Input: part model. Units: mm. Frame: model coordinates. Face numbers are marked on the shaded views. Give positions to 0.01 mm unless a question says otherwise; leave off trailing zeros. Loops run counter-clockwise (first coordinate to the right, second up) from the corner with the lowest first, then second, coordinate; pieces in that order, holes last. Notation, with made-up numbers: (47, 78) - (97, 78) arc R10 ccw to (97, 96) - close; hole circle Ø2 at (-15.75, 59.25). An arc over 180 degrees is marked (long way). Answer as a JSON object with one key per item and string values. Group by question number.
(1) Section query C-C (z = 12.95). Return loops of the section in (x, y).
(2) Pin query (flat end, axial travel): P1, Ø1.8, axis at y = 44.5, z = 11.5, coming from the +X side; P2, Ø3, axis at x = -43.5, z = 13, coming from the -Y side; P3, Ø20.5, axis at x = -19, y = 15.5, coming from the +Z side; P4, Ø3, axis at x = 3, z = 12.5, coming from the +Y side. Return the tip coordinate at first contact, or that it passes through.
(3) Material intervals for L1, parallel to Y at x = -15, z = 10.5; L2, parallel to Y at x = -17.5, z = 11.85; L3, parallel to X at y = 24, z = 10.9, sorted ascending.
(4) Section query B-B (y = 28.5). Return loops of the section in (x, z), plus the area to 3 significant figures.
(5) Section query D-D (y = 40.5). Return loops of the section in (x, z) (3 decimals), plus the area to 3 significant figures.
(6) Section query A-A (x = -22). Return loops of the section in (y, z), plus the area to 3 significant figures.
(7) Mould query, pull axis Y, two halves, no side actions, for the marked faces 1, 2 and 3. Classes: +Y half, -Y half, draft (parallel to the pull), parting line (faces both ways), or undercut.
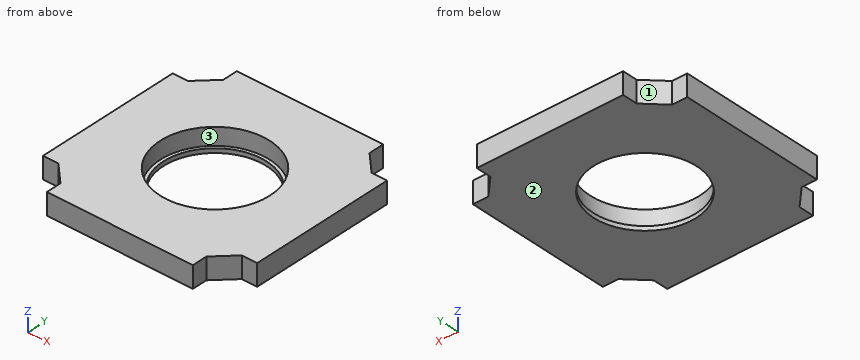
Autodesk Inventor part; units mm, degrees
ref_plane "Work Plane1" through (0, 0, 10) normal (0, 0, 1) x (1, 0, 0)
ref_plane "YZ Plane" through (0, 0, 0) normal (1, 0, 0) x (0, 1, 0)
ref_plane "XZ Plane" through (0, 0, 0) normal (0, 1, 0) x (-1, 0, 0)
ref_plane "Work Plane1" through (0, 0, 10) normal (0, 0, 1) x (1, 0, 0)
sketch "Sketch1" plane through (0, 0, 10) normal (0, 0, 1) x (1, 0, 0)
  line L0 (-4.0299, -0.3538) -> (-2.2322, 1.4439) construction
  arc A0 (-1.4439, 2.2322) -> (-2.2322, 1.4439) centre (-0.9299, 0.9299) ccw construction
  line L1 (-1.4439, 2.2322) -> (0.3538, 4.0299) construction
  line L2 (-37.8299, 42.8299) -> (-37.8299, 37.8299) construction
  line L3 (-37.8299, 37.8299) -> (-42.9208, 37.8299) construction
  line L4 (-37.8299, 42.2137) -> (-37.8299, 45.8299) construction
  line L5 (-37.8299, 45.8299) -> (-4.0299, 45.8299) construction
  line L6 (-4.0299, 45.8299) -> (-4.0299, 42.2137) construction
  line L7 (-4.0299, 4.0299) -> (0.3538, 4.0299)
  circle A1 centre (-20.9299, 20.9299) radius 17.5
  line L8 (-20.9299, 58.9723) -> (17.1124, 20.9299) construction
  line L9 (17.1124, 20.9299) -> (-20.9299, -17.1124) construction
  line L10 (-20.9299, -17.1124) -> (-58.9723, 20.9299) construction
  line L11 (-58.9723, 20.9299) -> (-20.9299, 58.9723) construction
  line L12 (-20.9299, 58.9723) -> (-20.9299, -17.1124) construction
  line L13 (17.1124, 20.9299) -> (-58.9723, 20.9299) construction
  line L14 (-20.9299, 58.9723) -> (32.8701, 58.9723) construction
  line L15 (-43.4299, 43.4299) -> (1.5701, 43.4299) construction
  line L16 (1.5701, 43.4299) -> (1.5701, -1.5701) construction
  line L17 (1.5701, -1.5701) -> (-43.4299, -1.5701) construction
  line L18 (-43.4299, -1.5701) -> (-43.4299, 43.4299) construction
  line L19 (-43.4299, 43.4299) -> (1.5701, -1.5701) construction
  line L20 (1.5701, 43.4299) -> (-43.4299, -1.5701) construction
  line L21 (-43.4299, 5.3876) -> (-43.4299, 36.4723)
  line L22 (-43.4299, 36.4723) -> (-36.4723, 43.4299)
  line L23 (-36.4723, 43.4299) -> (-5.3876, 43.4299)
  line L24 (-5.3876, 43.4299) -> (1.5701, 36.4723)
  line L25 (1.5701, 36.4723) -> (1.5701, 5.3876)
  line L26 (1.5701, 5.3876) -> (-5.3876, -1.5701)
  line L27 (-5.3876, -1.5701) -> (-36.4723, -1.5701)
  line L28 (-36.4723, -1.5701) -> (-43.4299, 5.3876)
  line L29 (-4.0299, 42.2137) -> (-37.8299, 42.2137)
  line L30 (-4.0299, -0.3538) -> (-4.0299, 4.0299)
  circle A2 centre (-20.9299, 20.9299) radius 1.5
  line L31 (-10.9299, 10.9299) -> (-30.9299, 10.9299) construction
  line L32 (-30.9299, 10.9299) -> (-30.9299, 30.9299) construction
  line L33 (-30.9299, 30.9299) -> (-10.9299, 30.9299) construction
  line L34 (-10.9299, 30.9299) -> (-10.9299, 10.9299) construction
  line L35 (-10.9299, 10.9299) -> (-30.9299, 30.9299) construction
  line L36 (-30.9299, 10.9299) -> (-10.9299, 30.9299) construction
  circle A3 centre (-30.9299, 30.9299) radius 1.4
  circle A4 centre (-30.9299, 10.9299) radius 1.4
  circle A5 centre (-10.9299, 10.9299) radius 1.4
  line L37 (-45.8299, 37.8299) -> (-42.0723, 37.8299) construction
  line L38 (-42.1723, 37.7299) -> (-45.8299, 37.7299)
  line L39 (-45.8299, 37.7299) -> (-45.8299, 4.1299)
  line L40 (-45.8299, 4.1299) -> (-42.1723, 4.1299)
  line L41 (-42.1723, 4.1299) -> (-42.1723, 37.7299)
  line L42 (-45.8299, 4.0299) -> (-42.0723, 4.0299) construction
  line L43 (-45.8299, 37.8299) -> (-42.0723, 37.8299)
  line L44 (-37.7299, 45.8299) -> (-4.1299, 45.8299)
  line L45 (-4.1299, 45.8299) -> (-4.1299, 42.1723)
  line L46 (-4.1299, 42.1723) -> (-37.7299, 42.1723)
  line L47 (-37.7299, 42.1723) -> (-37.7299, 45.8299)
  line L48 (0.4701, 37.8299) -> (0.4701, 4.0299) construction
  line L49 (0.4701, 4.0299) -> (3.9701, 4.0299) construction
  line L50 (3.9701, 37.8299) -> (3.9701, 4.0299) construction
  line L51 (0.4701, 37.8299) -> (3.9701, 37.8299) construction
  line L52 (-45.8299, -3.9701) -> (-4.0299, -3.9701) construction
  line L53 (0.3124, 37.7299) -> (3.9701, 37.7299)
  line L54 (3.9701, 37.7299) -> (3.9701, 4.1299)
  line L55 (3.9701, 4.1299) -> (0.3124, 4.1299)
  line L56 (0.3124, 4.1299) -> (0.3124, 37.7299)
  line L57 (-4.1713, -0.3538) -> (-37.7299, -0.3538)
  line L58 (-37.7299, -0.3538) -> (-37.7299, -3.9701)
  line L59 (-37.7299, -3.9701) -> (-4.1713, -3.9701)
  line L60 (-4.1713, -3.9701) -> (-4.1713, -0.3538)
  point P0 (-37.8299, 4.0299)
  dimension "d18" = 53.8
  dimension "d19" = 45
  dimension "d20" = 53.8
  dimension "d21" = 45
  dimension "d22" = 45
  dimension "d30" = 20
  dimension "d31" = 20
  dimension "d32" = 2.8
  dimension "d33" = 2.8
  dimension "d34" = 2.8
  dimension "d35" = 3
  dimension "d36" = 0.1
  dimension "d37" = 0.1
  dimension "d38" = 0.1
  dimension "d39" = 0.1
extrude "Extrusion1" add sketch "Sketch1" along normal blind 5 contours L30 L26 L57 L28 L41 L22 L46 L24 L56 L7 | L7 L26 L30 | L56 L24 L25 L26 | L26 L25 L24 L53 L54 L55 | L60 L59 L58 L57 L28 L27 L26 | L26 L27 L28 L57 | L46 L22 L29 L24 | L24 L29 L45 | L40 L39 L38 L22 L21 L28 | L28 L21 L22 L41 | L29 L22 L23 L24 | L24 L23 L22 L29 L47 L44 L45 | L47 L29 L22 | A1 | A2 | A3 | A4 | A5
sketch "Skizze4" plane through (0, 0, 15) normal (0, 0, 1) x (1, 0, 0)
  line L0 (-37.7299, 42.1723) -> (-42.1723, 37.7299)
  line L1 (-42.1723, 37.7299) -> (-45.8299, 37.7299)
  line L2 (-45.8299, 37.7299) -> (-45.8299, 4.1299) construction
  line L3 (-45.8299, 4.1299) -> (-42.1723, 4.1299)
  line L4 (-42.1723, 4.1299) -> (-37.6885, -0.3538)
  line L5 (-37.6885, -0.3538) -> (-37.7299, -0.3538)
  line L6 (-37.7299, -0.3538) -> (-37.7299, -3.9701)
  line L7 (-37.7299, -3.9701) -> (-4.1713, -3.9701) construction
  line L8 (-4.1713, -3.9701) -> (-4.1713, -0.3538)
  line L9 (-4.1713, -0.3538) -> (0.3124, 4.1299)
  line L10 (0.3124, 4.1299) -> (3.9701, 4.1299)
  line L11 (3.9701, 4.1299) -> (3.9701, 37.7299) construction
  line L12 (3.9701, 37.7299) -> (0.3124, 37.7299)
  line L13 (0.3124, 37.7299) -> (-4.1299, 42.1723)
  line L14 (-4.1299, 42.1723) -> (-4.1299, 45.8299)
  line L15 (-4.1299, 45.8299) -> (-37.7299, 45.8299) construction
  line L16 (-37.7299, 45.8299) -> (-37.7299, 42.1723)
  line L17 (-37.9299, 46.0299) -> (-3.9299, 46.0299) construction
  line L18 (-3.9299, 46.0299) -> (-3.9299, 42.2551)
  line L19 (-3.9299, 42.2551) -> (0.3953, 37.9299)
  line L20 (0.3953, 37.9299) -> (4.1701, 37.9299)
  line L21 (4.1701, 37.9299) -> (4.1701, 3.9299) construction
  line L22 (4.1701, 3.9299) -> (0.3953, 3.9299)
  line L23 (0.3953, 3.9299) -> (-3.9713, -0.4367)
  line L24 (-3.9713, -0.4367) -> (-3.9713, -4.1701)
  line L25 (-3.9713, -4.1701) -> (-37.9299, -4.1701) construction
  line L26 (-37.9299, -4.1701) -> (-37.9299, -0.3953)
  line L27 (-37.9299, -0.3953) -> (-42.2551, 3.9299)
  line L28 (-42.2551, 3.9299) -> (-46.0299, 3.9299)
  line L29 (-46.0299, 3.9299) -> (-46.0299, 37.9299) construction
  line L30 (-46.0299, 37.9299) -> (-42.2551, 37.9299)
  line L31 (-42.2551, 37.9299) -> (-37.9299, 42.2551)
  line L32 (-37.9299, 42.2551) -> (-37.9299, 46.0299)
  line L33 (-45.8299, 37.7299) -> (-45.8299, 37.9299)
  line L34 (-4.1299, 45.8299) -> (-37.7299, 45.8299)
  line L35 (-37.7299, 45.8299) -> (-37.9299, 45.8299)
  line L36 (-4.1299, 45.8299) -> (-3.9299, 45.8299)
  line L37 (3.9701, 37.7299) -> (3.9701, 37.9299)
  line L38 (3.9701, 4.1299) -> (3.9701, 37.7299)
  line L39 (3.9701, 4.1299) -> (3.9701, 3.9299)
  line L40 (-4.1713, -3.9701) -> (-3.9713, -3.9701)
  line L41 (-37.7299, -3.9701) -> (-37.9299, -3.9701)
  line L42 (-45.8299, 4.1299) -> (-45.8299, 3.9299)
  point P0 (0, 0)
  dimension "d40" = 0.2
extrude "IM_offset" add sketch "Skizze4" against normal up to surface (5 mm away)
sketch "Sketch20" plane through (0, 0, 15) normal (0, 0, 1) x (1, 0, 0)
  line L0 (-3.9299, 45.8299) -> (-37.9299, 45.8299)
  line L1 (-37.9299, 45.8299) -> (-37.9299, 42.2551)
  line L2 (-37.9299, 42.2551) -> (-42.2551, 37.9299)
  line L3 (-42.2551, 37.9299) -> (-45.8299, 37.9299)
  line L4 (-45.8299, 37.9299) -> (-45.8299, 3.9299)
  line L5 (-42.2551, 3.9299) -> (-45.8299, 3.9299)
  line L6 (-37.9299, -0.3953) -> (-42.2551, 3.9299)
  line L7 (-37.9299, -3.9701) -> (-37.9299, -0.3953)
  line L8 (-3.9713, -3.9701) -> (-37.9299, -3.9701)
  line L9 (-3.9713, -3.9701) -> (-3.9713, -0.4367)
  line L10 (-3.9713, -0.4367) -> (0.3953, 3.9299)
  line L11 (0.3953, 3.9299) -> (3.9701, 3.9299)
  line L12 (3.9701, 3.9299) -> (3.9701, 37.9299)
  line L13 (3.9701, 37.9299) -> (0.3953, 37.9299)
  line L14 (0.3953, 37.9299) -> (-3.9299, 42.2551)
  line L15 (-3.9299, 42.2551) -> (-3.9299, 45.8299)
  circle A0 centre (-20.9299, 20.9299) radius 12
  circle A1 centre (-28.9299, 12.9299) radius 3.95
  line L16 (-12.9299, 28.9299) -> (-28.9299, 28.9299)
  line L17 (-28.9299, 28.9299) -> (-28.9299, 12.9299)
  line L18 (-28.9299, 12.9299) -> (-12.9299, 12.9299)
  line L19 (-12.9299, 12.9299) -> (-12.9299, 28.9299)
  line L20 (-12.9299, 28.9299) -> (-28.9299, 12.9299) construction
  line L21 (-28.9299, 28.9299) -> (-12.9299, 12.9299) construction
  circle A2 centre (-28.9299, 28.9299) radius 3.95
  circle A3 centre (-12.9299, 28.9299) radius 3.95
  circle A4 centre (-12.9299, 12.9299) radius 3.95
  point P0 (0, 0)
  dimension "d113" = 24
  dimension "d114" = 7.9
  dimension "d115" = 16
  dimension "d116" = 16
  dimension "d117" = 7.9
  dimension "d118" = 7.9
  dimension "d119" = 7.9
extrude "Extrusion18" cut sketch "Sketch20" against normal through all contours A0 A4 L19 A3 | A3 L19 L16 A0 | A0 A4 L18 L19 | A3 L16 A2 A0 | A3 L16 L19 | L19 A4 L18 A1 L17 A2 L16 A3 | A0 A1 L18 A4 | L19 L18 A4 | A2 L16 L17 A0 | A0 A1 L17 L18 | A2 L17 A1 A0 | A2 L17 L16 | L18 L17 A1
sketch "Sketch23" plane through (0, 0, 15) normal (0, 0, 1) x (1, 0, 0)
  circle A0 centre (-20.9299, 20.9299) radius 12
  circle A1 centre (-20.9299, 20.9299) radius 12.75
  point P0 (0, 0)
  dimension "d140" = 25.5
extrude "Extrusion19" cut sketch "Sketch23" against normal blind 4
properties part number "20_Cube_Insert_Filter_25mm"
Recorded:
{
 "1": {"outline": "(-45.83, 3.93) - (-42.26, 3.93) - (-37.93, -0.4) - (-37.93, -3.97) - (-3.97, -3.97) - (-3.97, -0.44) - (0.4, 3.93) - (3.97, 3.93) - (3.97, 37.93) - (0.4, 37.93) - (-3.93, 42.26) - (-3.93, 45.83) - (-37.93, 45.83) - (-37.93, 42.26) - (-42.26, 37.93) - (-45.83, 37.93) - close; hole circle Ø25.5 at (-20.93, 20.93)"},
 "2": {"P1": "stops at x = -3.93", "P2": "stops at y = 3.67", "P3": "stops at z = 15", "P4": "stops at y = 37.93"},
 "3": {"L1": "y = -3.97 to 10.5, 31.36 to 45.83", "L2": "y = -3.97 to 8.65, 33.21 to 45.83", "L3": "x = -45.83 to -32.53, -9.33 to 3.97"},
 "4": {"outline": "(-45.83, 10) - (-30.24, 10) - (-30.24, 11) - (-31.19, 11) - (-31.19, 15) - (-45.83, 15) - close; (-11.62, 10) - (3.97, 10) - (3.97, 15) - (-10.67, 15) - (-10.67, 11) - (-11.62, 11) - close", "area": "148 mm^2"},
 "5": {"outline": "(-39.685, 10) - (-2.175, 10) - (-2.175, 15) - (-39.685, 15) - close", "area": "188 mm^2"},
 "6": {"outline": "(-3.97, 10) - (8.98, 10) - (8.98, 11) - (8.22, 11) - (8.22, 15) - (-3.97, 15) - close; (32.88, 10) - (45.83, 10) - (45.83, 15) - (33.63, 15) - (33.63, 11) - (32.88, 11) - close", "area": "123 mm^2"},
 "7": {"face 1": "+Y half", "face 2": "draft", "face 3": "undercut"}
}
